from build123d import *

# Parameters (mm, degrees)
SKETCH2_W             = 10
SKETCH2_H             = 20
BOSS_EXTRUDE1_DEPTH   = 15
SKETCH3_W             = 4.1
SKETCH3_H             = 10.1
CUT_EXTRUDE1_DEPTH    = 19.708286934
SKETCH4_W             = 2.95
SKETCH4_H             = 4.95
CUT_EXTRUDE2_DEPTH    = 15
SKETCH6_W             = 20
SKETCH6_H             = 15
BOSS_EXTRUDE2_DEPTH   = 3
BOSS_EXTRUDE3_DEPTH   = 5
CUT_EXTRUDE3_DEPTH    = 27.944433562
CUT_EXTRUDE4_DEPTH    = 0.5
BOSS_EXTRUDE6_START   = -10
BOSS_EXTRUDE6_DEPTH   = 20
BOSS_EXTRUDE6_2_DEPTH = 4.95
BOSS_EXTRUDE6_START_2 = 5.05
BOSS_EXTRUDE6_3_DEPTH = 4.95
BOSS_EXTRUDE6_4_DEPTH = 3
BOSS_EXTRUDE6_START_3 = 7
BOSS_EXTRUDE6_5_DEPTH = 3
BOSS_EXTRUDE6_6_DEPTH = 1
BOSS_EXTRUDE6_START_4 = -8
BOSS_EXTRUDE6_7_DEPTH = 1
BOSS_EXTRUDE6_8_DEPTH = 1
BOSS_EXTRUDE6_START_5 = 9
BOSS_EXTRUDE6_9_DEPTH = 1


# Read off the part's stored shape, not the designer's step: Boss-Extrude6
with BuildPart() as part:
    # Sketch2 → Boss-Extrude1 (new body)
    with BuildSketch(Plane(origin=(0, 0, 0), x_dir=(1, 0, 0), z_dir=(0, 1, 0))):
        Rectangle(SKETCH2_W, SKETCH2_H)
    extrude(amount=BOSS_EXTRUDE1_DEPTH)

    # Sketch3 → Cut-Extrude1 (cut, through all)
    with BuildSketch(Plane(origin=(0, 15, 0), x_dir=(1, 0, 0), z_dir=(0, 1, 0))):
        Rectangle(SKETCH3_W, SKETCH3_H)
    extrude(amount=-CUT_EXTRUDE1_DEPTH, mode=Mode.SUBTRACT)

    # Sketch4 → Cut-Extrude2 (cut)
    with BuildSketch(Plane(origin=(0, 15, 0), x_dir=(1, 0, 0), z_dir=(0, 1, 0))):
        Polygon((-2.05, 10), (-5, 10), (-5, -5.05), (-2.05, -5.05), (-2.05, 5.05), align=None)
        with Locations((-3.525, -7.525)):
            Rectangle(SKETCH4_W, SKETCH4_H)
    extrude(amount=-CUT_EXTRUDE2_DEPTH, mode=Mode.SUBTRACT)

    # Sketch6 → Boss-Extrude2 (add)
    with BuildSketch(Plane.ZY.offset(2.05)):
        with Locations((0, 7.5)):
            Rectangle(SKETCH6_W, SKETCH6_H)
    extrude(amount=BOSS_EXTRUDE2_DEPTH)

    # Sketch8 → Boss-Extrude3 (add)
    with BuildSketch(Plane.ZY.offset(5.05)):
        Polygon((-7, 15), (-10, 15), (-10, 0), (10, 0), (10, 15), (7, 15), (7, 3), (-7, 3), align=None)
    extrude(amount=BOSS_EXTRUDE3_DEPTH)

    # Sketch10 → Cut-Extrude3 (cut, through all)
    with BuildSketch(Plane.XY.offset(10)):
        Polygon((-10.05, 0), (5, 8.689121551), (5, 0), align=None)
    extrude(amount=-CUT_EXTRUDE3_DEPTH, mode=Mode.SUBTRACT)

    # Sketch11 → Cut-Extrude4 (cut)
    with BuildSketch(Plane.ZY.offset(10.05)):
        Polygon((-8, 2), (-8, 15), (-9, 15), (-9, 1), (0, 1), (9, 1), (9, 15), (8, 15), (8, 2), (0, 2), align=None)
    extrude(amount=-CUT_EXTRUDE4_DEPTH, mode=Mode.SUBTRACT)

    # Boss-Extrude6 outline → Boss-Extrude6 (add)
    with BuildSketch(Plane.XY.offset(BOSS_EXTRUDE6_START)):
        Polygon((-5.05, 17.886751346), (-5.05, 15), (-2.05, 15), (-2.05, 19.618802154), align=None)
        Polygon((2.05, 21.985938257), (2.05, 15), (5, 15), (5, 23.689121551), align=None)
    extrude(amount=BOSS_EXTRUDE6_DEPTH)

    # Boss-Extrude6 2 outline → Boss-Extrude6 2 (add)
    with BuildSketch(Plane.XY.offset(BOSS_EXTRUDE6_START)):
        Polygon((-2.05, 19.618802154), (-2.05, 15), (2.05, 15), (2.05, 21.985938257), align=None)
    extrude(amount=BOSS_EXTRUDE6_2_DEPTH)

    # Boss-Extrude6 3 outline → Boss-Extrude6 3 (add)
    with BuildSketch(Plane.XY.offset(BOSS_EXTRUDE6_START_2)):
        Polygon((-2.05, 19.618802154), (-2.05, 15), (2.05, 15), (2.05, 21.985938257), align=None)
    extrude(amount=BOSS_EXTRUDE6_3_DEPTH)

    # Boss-Extrude6 4 outline → Boss-Extrude6 4 (add)
    with BuildSketch(Plane.XY.offset(BOSS_EXTRUDE6_START)):
        Polygon((-9.55, 15), (-5.05, 15), (-5.05, 17.886751346), (-9.55, 15.288675135), align=None)
    extrude(amount=BOSS_EXTRUDE6_4_DEPTH)

    # Boss-Extrude6 5 outline → Boss-Extrude6 5 (add)
    with BuildSketch(Plane.XY.offset(BOSS_EXTRUDE6_START_3)):
        Polygon((-9.55, 15), (-5.05, 15), (-5.05, 17.886751346), (-9.55, 15.288675135), align=None)
    extrude(amount=BOSS_EXTRUDE6_5_DEPTH)

    # Boss-Extrude6 6 outline → Boss-Extrude6 6 (add)
    with BuildSketch(Plane.XY.offset(BOSS_EXTRUDE6_START)):
        Polygon((-10.05, 15), (-9.55, 15), (-9.55, 15.288675135), align=None)
    extrude(amount=BOSS_EXTRUDE6_6_DEPTH)

    # Boss-Extrude6 7 outline → Boss-Extrude6 7 (add)
    with BuildSketch(Plane.XY.offset(BOSS_EXTRUDE6_START_4)):
        Polygon((-10.05, 15), (-9.55, 15), (-9.55, 15.288675135), align=None)
    extrude(amount=BOSS_EXTRUDE6_7_DEPTH)

    # Boss-Extrude6 8 outline → Boss-Extrude6 8 (add)
    with BuildSketch(Plane.XY.offset(BOSS_EXTRUDE6_START_3)):
        Polygon((-10.05, 15), (-9.55, 15), (-9.55, 15.288675135), align=None)
    extrude(amount=BOSS_EXTRUDE6_8_DEPTH)

    # Boss-Extrude6 9 outline → Boss-Extrude6 9 (add)
    with BuildSketch(Plane.XY.offset(BOSS_EXTRUDE6_START_5)):
        Polygon((-10.05, 15), (-9.55, 15), (-9.55, 15.288675135), align=None)
    extrude(amount=BOSS_EXTRUDE6_9_DEPTH)


solid = part.part
Geometry check sheet. Reference: the model listing, model coordinates, mm. A direction names the side the tool comes from. Coordinates: 2 decimals unless noted, no trailing zeros. Order: outer loops, then holes, each group sorted by start corner. A loop starts at its lowest first (then second) coordinate and runs counter-clockwise, first axis right, second up. Notation, with made-up numbers: (3, -37.5) -> (46, -37.5) arc R12 cw to (46, -27.5) -> close; hole circle Ø5 at (11, -31.5). An arc over 180 degrees is marked (long way). Use a Markdown table: item, result. Add a question column.
1. Go/stop test with flat-tipped pins: pin 1 Ø3 at (x, z) = (1, -1) entering from -Y; pin 2 Ø4.5 at (y, z) = (10.5, -3) entering from -X; pin 3 Ø8 at (x, z) = (-4.5, 6) entering from +Y. Record where each tip stops, or that it passes through.
2. Cross-section at A-A (z = 0.75). Enter the section's corners in (x, y), and give its area (3 significant figures).
3. Material ranges on L1, parallel to Z at x = 1.25, y = 15.25; L2, parallel to X at y = 13.25, z = 1; L3, parallel to Z at x = -6.75, y = 16, recorded low to high.
4. Mould release check, pull along Z, two halves, no side actions. Record for faces 1 (the face through (-3, 12, -10)), 2 (the face through (-10.05, 0.3, -0.8)), 3 (the face through (-2.05, 12, 0)): pulls with the +Z half, pulls with the -Z half, needs draft (parallel to the pull), parting line crosses it, or undercut.
5. Cross-section at B-B (y = 9). Enter the section's corners in (x, z).
6. Cross-section at D-D (z = 7.5). Enter the section's corners in (x, y).
7. Cross-section at C-C (x = 0.5). Enter the section's corners in (y, z).
8. Set-up check for faces 4 (the face through (-3, 12, 10)), 5 (the face through (-8, 11, -7)), 6 (the face through (0, 13, -5.05)): record each of +Z, -Z, +X, -X, +Y, -Y from which the full face is reachable in a straight line by a thin tool's end or side.
Filled sheet:
| question | item | result |
|---|---|---|
| 1 | pin 1 | y = 6.99 |
| 1 | pin 2 | x = -5.05 |
| 1 | pin 3 | y = 20.51 |
| 2 | outline | (-10.05, 0) -> (-2.05, 4.62) -> (-2.05, 19.62) -> (-5.05, 17.89) -> (-5.05, 3) -> (-10.05, 3) -> (-10.05, 2) -> (-9.55, 2) -> (-9.55, 1) -> (-10.05, 1) -> close; (2.05, 6.99) -> (5, 8.69) -> (5, 23.69) -> (2.05, 21.99) -> close |
| 2 | area | 96.5 mm2 |
| 3 | L1 | -10 to -5.05, 5.05 to 10 |
| 3 | L2 | -5.05 to -2.05, 2.05 to 5 |
| 3 | L3 | -10 to -7, 7 to 10 |
| 4 | face 1 | pulls with the -Z half |
| 4 | face 2 | needs draft |
| 4 | face 3 | undercut |
| 5 | outline | (-10.05, -10) -> (5, -10) -> (5, 10) -> (-10.05, 10) -> (-10.05, 9) -> (-9.55, 9) -> (-9.55, 8) -> (-10.05, 8) -> (-10.05, 7) -> (-5.05, 7) -> (-5.05, -7) -> (-10.05, -7) -> (-10.05, -8) -> (-9.55, -8) -> (-9.55, -9) -> (-10.05, -9) -> close; hole (-2.05, -5.05) -> (2.05, -5.05) -> (2.05, 5.05) -> (-2.05, 5.05) -> close |
| 6 | outline | (-10.05, 0) -> (5, 8.69) -> (5, 23.69) -> (-10.05, 15) -> (-10.05, 2) -> (-9.55, 2) -> (-9.55, 1) -> (-10.05, 1) -> close |
| 7 | outline | (6.09, -10) -> (21.09, -10) -> (21.09, -5.05) -> (6.09, -5.05) -> close; (6.09, 5.05) -> (21.09, 5.05) -> (21.09, 10) -> (6.09, 10) -> close |
| 8 | face 4 | +Z, +X, -X, +Y, -Y |
| 8 | face 5 | -X, +Y |
| 8 | face 6 | +Y, -Y |
